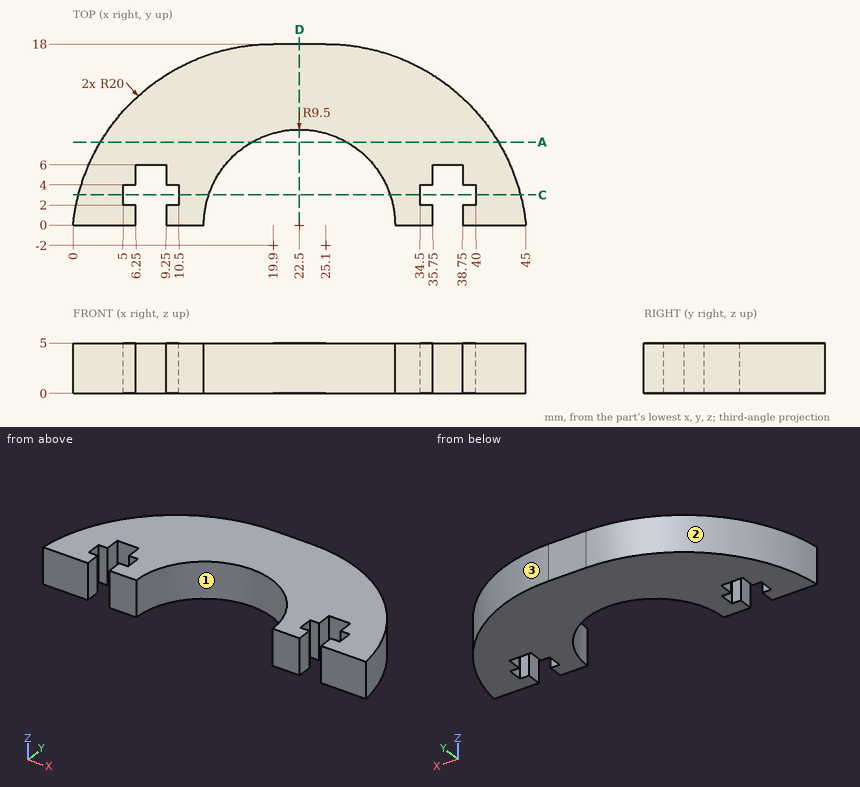
Input: dimensioned drawing with shaded views. Units: mm. Origin: part minimum x, y, z. Coordinates: 2 decimals unless noted, no trailing zeros. Order: outer loops, then holes, each group sorted by start corner. A loop starts at its lowest first (then second) coordinate and runs counter-clockwise, first axis right, second up.
(1) Section query A-A (y = 8.25). Return the cut outline in (x, z).
(2) Section query D-D (x = 22.5). Return the cut outline in (y, z).
(3) Draft query along X for the marked faces 1, 2 and 3. Return one class per face: pulls with the +X half, pulls with the -X half, needs draft (parallel to the pull), parting line crosses it, or undercut.
(4) Section query C-C (y = 3). Return the cut outline in (x, z) (1 decimal), plus the area to 3 significant figures.
(5) Material intervals for probe 1 along X at (y, z) = (2.75, 1.1); probe 2 along X at (y, z) = (1, 3); probe 3 along X at (y, z) = (7.75, 3.9) (1 decimal), sorted ascending.
(6) First-contact query: pin 1 (2 mm diameter, centred on y = 3, z = 3, fed in from -X); pin 2 (2 mm diameter, centred on y = 5.5, z = 2, fed in from +X) (1 decimal); pin 3 (1.6 mm diameter, centred on y = 5, z = 3, fed in from -X) (1 decimal). Flat tips, straight axial feed; report the tip coordinate or a pass-through.
Solution:
1. outline: (2.73, 0) - (17.79, 0) - (17.79, 5) - (2.73, 5) - close; (27.21, 0) - (42.27, 0) - (42.27, 5) - (27.21, 5) - close
2. outline: (9.5, 0) - (18, 0) - (18, 5) - (9.5, 5) - close
3. face 1: undercut
3. face 2: pulls with the -X half
3. face 3: pulls with the +X half
4. outline: (0.5, 0) - (5, 0) - (5, 5) - (0.5, 5) - close; (10.5, 0) - (13.5, 0) - (13.5, 5) - (10.5, 5) - close; (31.5, 0) - (34.5, 0) - (34.5, 5) - (31.5, 5) - close; (40, 0) - (44.5, 0) - (44.5, 5) - (40, 5) - close
4. area: 74.5 mm2
5. probe 1: x = 0.47 to 5, 10.5 to 13.41, 31.59 to 34.5, 40 to 44.53
5. probe 2: x = 0.13 to 6.25, 9.25 to 13.05, 31.95 to 35.75, 38.75 to 44.87
5. probe 3: x = 2.4 to 17, 28 to 42.6
6. pin 1: stops at x = 0.3
6. pin 2: stops at x = 44
6. pin 3: stops at x = 0.9
